from build123d import *

# Parameters (mm, degrees)
SKETCH_1_R          = 1.6
SKETCH_1_W          = 30
SKETCH_1_H          = 13
EXTRUDE_1_DEPTH     = 10
SKETCH_2_R          = 1.65
CUT_EXTRUDE_1_DEPTH = 54.632918996
SKETCH_4_R          = 3
CUT_EXTRUDE_3_DEPTH = 5
SKETCH_6_W          = 80
SKETCH_6_H          = 2
CUT_EXTRUDE_5_DEPTH = 45.655598753
FILLET_1_R          = 3


with BuildPart() as part:
    # 草图1 → 凸台-拉伸1 (new body)
    with BuildSketch(Plane(origin=(0, 0, 0), x_dir=(1, 0, 0), z_dir=(0, 1, 0))):
        Polygon((-40, -17.15), (-40, 17.15), (40, 17.15), (40, -17.15), (20, -17.15), (-20, -17.15), align=None)
        with Locations(Location((-35, 11.65, 0), (0, 0, 270))):
            Circle(SKETCH_1_R, mode=Mode.SUBTRACT)
        with Locations(Location((-35, -11.35, 0), (0, 0, 270))):
            Circle(SKETCH_1_R, mode=Mode.SUBTRACT)
        with Locations(Location((35, -11.35, 0), (0, 0, 90))):
            Circle(SKETCH_1_R, mode=Mode.SUBTRACT)
        with Locations(Location((35, 11.65, 0), (0, 0, 90))):
            Circle(SKETCH_1_R, mode=Mode.SUBTRACT)
        with Locations((-20, 0)):
            Rectangle(SKETCH_1_W, SKETCH_1_H, mode=Mode.SUBTRACT)
        with Locations((20, 0)):
            Rectangle(SKETCH_1_W, SKETCH_1_H, mode=Mode.SUBTRACT)
    extrude(amount=EXTRUDE_1_DEPTH)

    # 草图2 → 切除-拉伸1 (cut, through all)
    with BuildSketch(Plane(origin=(0, 0, -17.15), x_dir=(-1, 0, 0), z_dir=(0, 0, -1))):
        with Locations((-20, 4.5)):
            Circle(SKETCH_2_R)
        with Locations(Location((20, 4.5, 0), (0, 0, 180))):
            Circle(SKETCH_2_R)
    extrude(amount=-CUT_EXTRUDE_1_DEPTH, mode=Mode.SUBTRACT)

    # 草图4 → 切除-拉伸3 (cut)
    with BuildSketch(Plane(origin=(0, 0, -17.15), x_dir=(-1, 0, 0), z_dir=(0, 0, -1))):
        with Locations((-20, 4.5)):
            Circle(SKETCH_4_R)
        with Locations(Location((20, 4.5, 0), (0, 0, 180))):
            Circle(SKETCH_4_R)
    extrude(amount=-CUT_EXTRUDE_3_DEPTH, mode=Mode.SUBTRACT)

    # 草图6 → 切除-拉伸5 (cut, through all)
    with BuildSketch(Plane(origin=(0, 10, 0), x_dir=(1, 0, 0), z_dir=(0, 1, 0))):
        with Locations((0, 16.15)):
            Rectangle(SKETCH_6_W, SKETCH_6_H)
    extrude(amount=-CUT_EXTRUDE_5_DEPTH, mode=Mode.SUBTRACT)

    # 圆角1
    fillet_1_edges = [part.edges().sort_by_distance(p)[0] for p in [
        (40, 5, -15.15),
        (-40, 5, -15.15),
        (40, 5, 17.15),
        (-40, 5, 17.15),
        (-35, 5, -6.5),
        (-35, 5, 6.5),
        (-5, 5, 6.5),
        (-5, 5, -6.5),
        (35, 5, -6.5),
        (5, 5, -6.5),
        (5, 5, 6.5),
        (35, 5, 6.5),
    ]]
    fillet(fillet_1_edges, radius=FILLET_1_R)


solid = part.part
Build history of the part. All positions in model axes, mm. A direction names the side the tool comes from. Give positions to 0.01 mm unless a question says otherwise; leave off trailing zeros. Order: outer loops, then holes, each group sorted by start corner. A loop starts at its lowest first (then second) coordinate and runs counter-clockwise, first axis right, second up. Notation, with made-up numbers: M 82,27 L 124,27 A13 cw 124,46 Z; hole C 60,13.25 d1. An arc over 180 degrees is marked long. Put each result on its own line as item: value.
Item 1: Cut at A-A on x = 20. Write the cut outline in (y, z), then the cut area to 3 significant figures.
Results are:
outline: M 0,-15.15 L 1.5,-15.15 L 1.5,-12.15 L 2.85,-12.15 L 2.85,-6.5 L 0,-6.5 Z; M 0,6.5 L 2.85,6.5 L 2.85,17.15 L 0,17.15 Z; M 6.15,-12.15 L 7.5,-12.15 L 7.5,-15.15 L 10,-15.15 L 10,-6.5 L 6.15,-6.5 Z; M 6.15,6.5 L 10,6.5 L 10,17.15 L 6.15,17.15 Z
area: 121 mm2
Item 2: Pull direction Z, two halves, no side cores. Call faces 1 (the face through (-39.14, 4.93, -14.25)), 2 (the face through (-1, 5, 17.15)), 3 (the face through (19.8, 2.7, -6.5)), 4 (the face through (34.1, 5.07, -5.64)): +Z half, -Z half, draft (parallel to the pull), parting line (faces both ways), or undercut.
Results are:
face 1: -Z half
face 2: +Z half
face 3: undercut
face 4: undercut
Item 3: Wall check: probe 1 along X at (y, z) = (0.75, -2); probe 2 along Z at (x, y) = (25, 2.5); probe 3 along X at (y, z) = (4, 15). Give the ranges that are in metal, low to high.
Results are:
probe 1: -40 to -35, -5 to 5, 35 to 40
probe 2: -15.15 to -6.5, 6.5 to 17.15
probe 3: -39.88 to -21.57, -18.43 to 18.43, 21.57 to 39.88
Item 4: Cut at B-B on z = 11.35. Write the cut outline in (x, y).
Results are:
outline: M -40,0 L -36.6,0 L -36.6,10 L -40,10 Z; M -33.4,0 L 33.4,0 L 33.4,10 L -33.4,10 Z; M 36.6,0 L 40,0 L 40,10 L 36.6,10 Z; hole C -20,4.5 d3.3; hole C 20,4.5 d3.3
Item 5: Which spindle directions (+Z, -Z, +X, -X, +Y, -Y) get a long thin tool onto all of the face, cutting with end or side? Do faces 5 (the face through (-21.31, 5.5, -9.36)), 6 (the face through (-34.14, 5.07, 5.6)), 7 (the face through (22.4, 2.7, -13.7)). Say none if no direction does.
Results are:
face 5: +Z, -Z
face 6: +Y, -Y
face 7: -Z
Item 6: Cut at C-C on y = 4.5. Count the separate pieces of the cut face and the enclosed holes in it, then the cut area to 3 significant figures.
Results are:
separate pieces: 3
enclosed holes: 4
area: 1,640 mm2
Item 7: Cut at D-D on x = 10. Write the cut outline in (y, z).
Results are:
outline: M 0,-15.15 L 10,-15.15 L 10,-6.5 L 0,-6.5 Z; M 0,6.5 L 10,6.5 L 10,17.15 L 0,17.15 Z
Item 8: Drop a flat-ended pin along its axis: pin 1 Ø3 at (x, y) = (-20, 3.5) entering from -Z. Give the stop position or say it passes through.
Results are:
pin 1: z = -12.15
